The model under review builds one solid part; all positions refer to its coordinate system, in mm. A direction names the side the tool comes from. Round coordinates to 2 decimals unless told otherwise and drop trailing zeros. Loops run counter-clockwise (first coordinate to the right, second up) from the corner with the lowest first, then second, coordinate; pieces in that order, holes last. Notation, with made-up numbers: (33, -17.75) - (54, -17.75) arc R26 cw to (54, -2.75) - close; hole circle Ø11 at (88.5, 87). An arc over 180 degrees is marked (long way). Answer as CSV lines item,"result".
from build123d import *

# Parameters (mm, degrees)
SKETCH_1_W               = 2
SKETCH_1_H               = 58
EXTRUDE_1_DEPTH          = 53
SKETCH_4_W               = 5
SKETCH_4_H               = 35
EXTRUDE_3_DEPTH          = 19.5
CUT_EXTRUDE_START        = -0.8
SKETCH_9_W               = 5
SKETCH_9_H               = 20
CUT_EXTRUDE_5_DEPTH      = 16.7
SKETCH_10_R              = 2
CUT_EXTRUDE_6_DEPTH      = 10
SKETCH_11_W              = 38.5
SKETCH_11_H              = 6
SKETCH_11_H_2            = 42
SKETCH_11_W_2            = 4.5
SKETCH_11_H_3            = 23
CUT_EXTRUDE_7_DEPTH      = 10
FILLET_1_R               = 5
EXTRUDE_4_DEPTH          = 35
EXTRUDE_5_DEPTH          = 35
CUT_EXTRUDE_START_2      = 5
SKETCH_14_W              = 17.67500243
SKETCH_14_H              = 173.36044852
CUT_EXTRUDE_9_DEPTH      = 12
CUT_EXTRUDE_START_3      = 19
CUT_EXTRUDE_10_DEPTH     = 18
SKETCH_16_W              = 19.32347426
SKETCH_16_H              = 7.4
SKETCH_16_W_2            = 22.441906264
SKETCH_16_H_2            = 6.4
CUT_EXTRUDE_11_DEPTH     = 10
CUT_EXTRUDE_8_DEPTH      = 20
CUT_EXTRUDE_8_DEPTH_BACK = 43


with BuildPart() as part:
    # Эскиз1 → Бобышка-Вытянуть1 (new body)
    with BuildSketch(Plane.XY):
        with Locations((1, -29)):
            Rectangle(SKETCH_1_W, SKETCH_1_H)
    extrude(amount=EXTRUDE_1_DEPTH)

    # Эскиз4 → Бобышка-Вытянуть3 (add)
    with BuildSketch(Plane.ZY):
        with Locations((2.5, -40.5)):
            Rectangle(SKETCH_4_W, SKETCH_4_H)
    extrude(amount=-EXTRUDE_3_DEPTH)

    # Эскиз9 → Вырез-Вытянуть5 (cut)
    with BuildSketch(Plane(origin=(19.5, 0, 0), x_dir=(0, 0, -1), z_dir=(1, 0, 0)).offset(CUT_EXTRUDE_START)):
        with Locations((-2.5, -41)):
            Rectangle(SKETCH_9_W, SKETCH_9_H)
    extrude(amount=-CUT_EXTRUDE_5_DEPTH, mode=Mode.SUBTRACT)

    # Эскиз10 → Вырез-Вытянуть6 (cut)
    with BuildSketch(Plane(origin=(2, 0, 0), x_dir=(0, 0, -1), z_dir=(1, 0, 0))):
        with Locations(Location((-48.5, -47, 0), (0, 0, 90))):
            Circle(SKETCH_10_R)
        with Locations(Location((-9.5, -4, 0), (0, 0, 90))):
            Circle(SKETCH_10_R)
    extrude(amount=-CUT_EXTRUDE_6_DEPTH, mode=Mode.SUBTRACT)

    # Эскиз11 → Вырез-Вытянуть7 (cut)
    with BuildSketch(Plane(origin=(2, 0, 0), x_dir=(0, 0, -1), z_dir=(1, 0, 0))):
        with Locations((-33.75, -55)):
            Rectangle(SKETCH_11_W, SKETCH_11_H)
        with Locations((-33.75, -21)):
            Rectangle(SKETCH_11_W, SKETCH_11_H_2)
        with Locations((-2.25, -11.5)):
            Rectangle(SKETCH_11_W_2, SKETCH_11_H_3)
    extrude(amount=-CUT_EXTRUDE_7_DEPTH, mode=Mode.SUBTRACT)

    # Скругление1
    fillet_1_edges = [part.edges().sort_by_distance(p)[0] for p in [
        (1, -42, 14.5),
        (1, 0, 4.5),
        (1, 0, 14.5),
        (1, -58, 14.5),
        (1, -42, 53),
        (1, -52, 53),
    ]]
    fillet(fillet_1_edges, radius=FILLET_1_R - 0.0001)  # a hair under: the kernel refuses the full size

    # Эскиз12 → Бобышка-Вытянуть4 (add)
    with BuildSketch(Plane.XZ.offset(58)):
        Polygon((0, 0), (0, 15), (-15, 15), align=None)
    extrude(amount=-EXTRUDE_4_DEPTH)

    # Эскиз13 → Бобышка-Вытянуть5 (add)
    with BuildSketch(Plane(origin=(0, -23, 0), x_dir=(1, 0, 0), z_dir=(0, 1, 0))):
        Polygon((0, 0), (19.5, 0), (19.5, 22.111293257), (12.772431149, 17.644276295), (12.772431149, 12.772431149), align=None)
    extrude(amount=-EXTRUDE_5_DEPTH)

    # Эскиз14 → Вырез-Вытянуть9 (cut)
    with BuildSketch(Plane.ZY.offset(-2).offset(CUT_EXTRUDE_START_2)):
        with Locations((6.192960349, -52.7238676)):
            Rectangle(SKETCH_14_W, SKETCH_14_H)
    extrude(amount=CUT_EXTRUDE_9_DEPTH, mode=Mode.SUBTRACT)

    # Эскиз15 → Вырез-Вытянуть10 (cut)
    with BuildSketch(Plane.XZ.offset(31).offset(CUT_EXTRUDE_START_3)):
        Polygon((18.1, 0), (14.172431149, 0), (14.172431149, -12.192532161), (14.172431149, -24.03140998), (18.1, -24.03140998), align=None)
        Polygon((14.172431149, -12.192532161), (14.172431149, 0), (2, 0), (1.979898987, 0), align=None)
    extrude(amount=-CUT_EXTRUDE_10_DEPTH, mode=Mode.SUBTRACT)

    # Эскиз16 → Вырез-Вытянуть11 (cut)
    with BuildSketch(Plane.ZY.offset(-12.772431149)):
        with Locations((-22.434168279, -26.7)):
            Rectangle(SKETCH_16_W, SKETCH_16_H)
        with Locations((-23.993384281, -54.8)):
            Rectangle(SKETCH_16_W_2, SKETCH_16_H_2)
    extrude(amount=-CUT_EXTRUDE_11_DEPTH, mode=Mode.SUBTRACT)

    # Эскиз8 → Вырез-Вытянуть8 (cut, two sides: drawn at the far end of the back side and taken through both)
    with BuildSketch(Plane(origin=(0, 0, 0), x_dir=(-0.7071067811865437, 0, -0.7071067811865515), z_dir=(0.7071067811865515, 0, -0.7071067811865437)).offset(-CUT_EXTRUDE_8_DEPTH_BACK)):
        with BuildLine():
            Line((-2, -29.25), (0, -29.25))
            Line((0, -29.25), (0, -27.75))
            Line((0, -27.75), (-1.133974596, -27.75))
            Line((-1.133974596, -27.75), (-1.700961894, -26.767949192))
            ThreePointArc((-1.700961894, -26.767949192), (-1.626036577, -26.948834909), (-1.600480947, -27.142949192))
            ThreePointArc((-1.600480947, -27.142949192), (-2.156366663, -27.867393562), (-3, -27.517949192))
            Line((-3, -27.517949192), (-2, -29.25))
        make_face()
        with BuildLine():
            ThreePointArc((-1.700961894, -26.767949192), (-2.725480947, -26.49343014), (-3, -27.517949192))
            Line((-3, -27.517949192), (-1.700961894, -26.767949192))
        make_face()
        with BuildLine():
            Line((-1.700961894, -26.767949192), (-3, -27.517949192))
            ThreePointArc((-3, -27.517949192), (-2.156366663, -27.867393562), (-1.600480947, -27.142949192))
            ThreePointArc((-1.600480947, -27.142949192), (-1.626036577, -26.948834909), (-1.700961894, -26.767949192))
        make_face()
        with BuildLine():
            ThreePointArc((-3, -53.482050808), (-2.725480947, -54.50656986), (-1.700961894, -54.232050808))
            Line((-1.700961894, -54.232050808), (-3, -53.482050808))
        make_face()
        with BuildLine():
            Line((-3, -53.482050808), (-1.700961894, -54.232050808))
            ThreePointArc((-1.700961894, -54.232050808), (-1.626036577, -54.051165091), (-1.600480947, -53.857050808))
            ThreePointArc((-1.600480947, -53.857050808), (-2.156366663, -53.132606438), (-3, -53.482050808))
        make_face()
        with BuildLine():
            Line((-1.133974596, -53.25), (0, -53.25))
            Line((0, -53.25), (0, -51.75))
            Line((0, -51.75), (-2, -51.75))
            Line((-2, -51.75), (-3, -53.482050808))
            ThreePointArc((-3, -53.482050808), (-2.156366663, -53.132606438), (-1.600480947, -53.857050808))
            ThreePointArc((-1.600480947, -53.857050808), (-1.626036577, -54.051165091), (-1.700961894, -54.232050808))
            Line((-1.700961894, -54.232050808), (-1.133974596, -53.25))
        make_face()
    extrude(amount=CUT_EXTRUDE_8_DEPTH + CUT_EXTRUDE_8_DEPTH_BACK, mode=Mode.SUBTRACT)


solid = part.part
1. Tool access review of faces 1 (the face through (14.172, -41, -15)), 2 (the face through (5, -29.25, -4)), 3 (the face through (-1, -41, 15)), 4 (the face through (7.99, -41.13, -6.01)): name each direction out of +Z, -Z, +X, -X, +Y, -Y from which nothing blocks a thin tool from reaching the whole face with its end or side.
Numbers:
face 1,"+Z, -Z"
face 2,"-Z, -X"
face 3,"+Z, -X, +Y, -Y"
face 4,"+Z"
2. Draft analysis for pull direction Y (two halves, no side actions). For faces 5 (the face through (0, -47, 34)), 6 (the face through (5.758, -27.266, -3.759)), 7 (the face through (16, -51.6, -16)), state which applies: +Y half, -Y half, draft (parallel to the pull), parting line (faces both ways), or undercut.
Numbers:
face 5,"draft"
face 6,"undercut"
face 7,"-Y half"
3. Take a section at D-D (y = -18.5). State the section outline as (x, z) points.
Numbers:
outline,"(0, 4.5) - (2, 4.5) - (2, 14.5) - (0, 14.5) - close"
4. Take a section at B-B (z = 31.5). State the section outline as (x, y) points.
Numbers:
outline,"(0, -52) - (2, -52) - (2, -42) - (0, -42) - close"
5. Wall thickness on probe 1 along X at (y, z) = (-44, -3); probe 2 along Y at (x, z) = (13.75, 2); probe 3 along Y at (x, z) = (0.75, 15): over which ranges is each line inside the solid? List them lowest first.
Numbers:
probe 1,"x = 3 to 4.98, 18.1 to 19.5"
probe 2,"y = -58 to -51, -31 to -23"
probe 3,"y = -52 to -39.18"
6. Take a section at C-C (y = -4). State the section outline as (x, z) points.
Numbers:
outline,"(0, 4.6) - (2, 4.6) - (2, 7.5) - (0, 7.5) - close; (0, 11.5) - (2, 11.5) - (2, 14.4) - (0, 14.4) - close"
7. Clearance check with flat-ended pins moving along their axes: pin 1 (9 mm diameter, centred on y = -44.5, z = -7.5, fed in from -X); pin 2 (8 mm diameter, centred on x = 6, z = -9, fed in from -Y); pin 3 (2 mm diameter, centred on x = 16, z = -18.5, fed in from -Y); pin 4 (2.5 mm diameter, centred on x = -2, y = -43.5, fed in from +Z). State where each tip first meets the part, or that it passes through.
Numbers:
pin 1,"stops at x = 3"
pin 2,"stops at y = -58"
pin 3,"stops at y = -51.6"
pin 4,"stops at z = 15"
